The listing builds one solid part. Answer for the finished solid, in the listing's coordinates (mm). Face numbers are marked on the shaded views. Give positions to 0.01 mm unless a question says otherwise; leave off trailing zeros. Loops run counter-clockwise (first coordinate to the right, second up) from the corner with the lowest first, then second, coordinate; pieces in that order, holes last. Notation, with made-up numbers: (55.5, 56.25) - (74.5, 56.25) arc R23 cw to (74.5, 74.25) - close; hole circle Ø10 at (-27.75, 57). An arc over 180 degrees is marked (long way). Write each question's results on one line, items separated by ' | '.
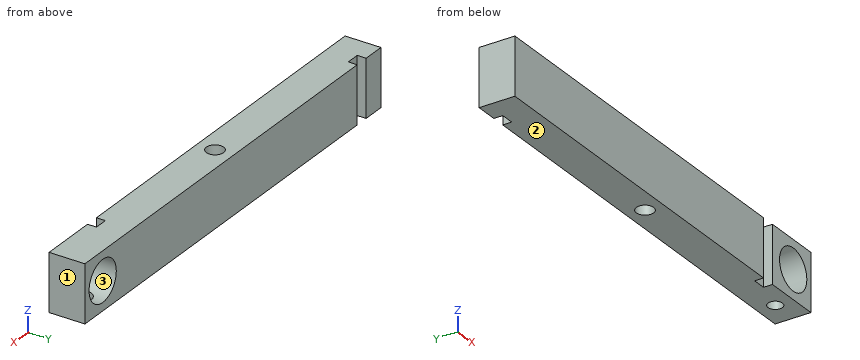
from build123d import *

# Parameters (mm, degrees)
SKETCH1_W                    = 127
SKETCH1_H                    = 10.16
BOSS_EXTRUDE1_DEPTH          = 8.128
F_10_0_1935_DIAMETER_HOLE2_D = 4.9149
SKETCH6_W                    = 3.81
SKETCH6_H                    = 2.54
CUT_EXTRUDE1_DEPTH           = 16.256
HOLE1_D                      = 11.684
HOLE2_D                      = 4.064
HOLE2_DEPTH                  = 6.906051222
HOLE2_TIP                    = 1.220948778


with BuildPart() as part:
    # Sketch1 → Boss-Extrude1 (new body, symmetric)
    with BuildSketch(Plane.XY):
        Rectangle(SKETCH1_W, SKETCH1_H)
    extrude(amount=BOSS_EXTRUDE1_DEPTH, both=True)

    # #10 (0.1935) Diameter Hole2 (through all)
    with Locations(Plane.XY.offset(8.128)):
        with Locations((0, 0)):
            Hole(F_10_0_1935_DIAMETER_HOLE2_D / 2)

    # Sketch6 → Cut-Extrude1 (cut)
    with BuildSketch(Plane.XY.offset(8.128)):
        with Locations((-55.245, 3.81)):
            Rectangle(SKETCH6_W, SKETCH6_H)
        with Locations((45.085, -3.81)):
            Rectangle(SKETCH6_W, SKETCH6_H)
    extrude(amount=-CUT_EXTRUDE1_DEPTH, mode=Mode.SUBTRACT)

    # Hole1 (through all)
    with Locations(Plane(origin=(0, 5.08, 0), x_dir=(1, 0, 0), z_dir=(0, 1, 0))):
        with Locations((55.88, 0)):
            Hole(HOLE1_D / 2)

    # Hole2
    with Locations(Plane(origin=(0, 0, -8.128), x_dir=(-1, 0, 0), z_dir=(0, 0, -1))):
        with Locations((-55.88, 0)):
            Hole(HOLE2_D / 2, depth=HOLE2_DEPTH)
            with Locations((0, 0, -(HOLE2_DEPTH + HOLE2_TIP / 2))):  # 118° drill point
                Cone(0, HOLE2_D / 2, HOLE2_TIP, mode=Mode.SUBTRACT)


solid = part.part
Item 1: A cutting plane is placed at D-D, the plane x = 55.88. Determine the outline of the cut face in (y, z), plus the area to 3 significant figures.
Values found:
outline: (-5.08, -8.13) - (-2.03, -8.13) - (-2.03, -5.84) - (-5.08, -5.84) - close; (-5.08, 5.84) - (5.08, 5.84) - (5.08, 8.13) - (-5.08, 8.13) - close; (2.03, -8.13) - (5.08, -8.13) - (5.08, -5.84) - (2.03, -5.84) - close | area: 37.2 mm²
Item 2: For a pull along Z with two mould halves and no side action, classify the marked faces 1, 2 and 3 as released by +Z, released by -Z, zero draft, split by the parting line, or undercut.
Values found:
face 1: zero draft | face 2: released by -Z | face 3: undercut
Item 3: A cutting plane is placed at C-C, the plane x = 0. Determine the outline of the cut face in (y, z), plus the area to 3 significant figures.
Values found:
outline: (-5.08, -8.13) - (-2.46, -8.13) - (-2.46, 8.13) - (-5.08, 8.13) - close; (2.46, -8.13) - (5.08, -8.13) - (5.08, 8.13) - (2.46, 8.13) - close | area: 85.3 mm²
Item 4: A cutting plane is placed at B-B, the plane y = -3.75. Determine the outline of the cut face in (x, z), plus the area to 3 significant figures.
Values found:
outline: (-63.5, -8.13) - (43.18, -8.13) - (43.18, 8.13) - (-63.5, 8.13) - close; (46.99, -8.13) - (63.5, -8.13) - (63.5, 8.13) - (46.99, 8.13) - close; hole circle Ø11.68 at (55.88, 0) | area: 1,900 mm²
Item 5: Find the intervals of material crossed by line 1 along X through (y, z) = (-4, -2.5); line 2 along Z through (x, y) = (55.88, 3); line 3 along Z through (x, y) = (55.88, -1), in increasing order. Write a range as [from, to].
Values found:
line 1: x = [-63.5, 43.18], [46.99, 50.6], [61.16, 63.5] | line 2: z = [-8.13, -5.84], [5.84, 8.13] | line 3: z = [5.84, 8.13]
Item 6: A flat-ended cylindrical pin translates along its axis: P1, Ø1.9, axis at x = -55.5, z = 1, coming from the +Y side. Find the tip coordinate at first contact, or state that the pin passes through.
Values found:
P1: stops at y = 2.54
Item 7: A cutting plane is placed at A-A, the plane z = 0. Determine the outline of the cut face in (x, y).
Values found:
outline: (-63.5, -5.08) - (43.18, -5.08) - (43.18, -2.54) - (46.99, -2.54) - (46.99, -5.08) - (50.04, -5.08) - (50.04, 5.08) - (-53.34, 5.08) - (-53.34, 2.54) - (-57.15, 2.54) - (-57.15, 5.08) - (-63.5, 5.08) - close; (61.72, -5.08) - (63.5, -5.08) - (63.5, 5.08) - (61.72, 5.08) - close; hole circle Ø4.91 at (0, 0)
